Check sheet for the modelled part. Datum: model origin and axes. Units: mm. A direction names the side the tool comes from. Coordinates: 2 decimals unless noted, no trailing zeros. Loops run counter-clockwise (first coordinate to the right, second up) from the corner with the lowest first, then second, coordinate; pieces in that order, holes last. Notation, with made-up numbers: (60, 7) -> (112, 7) arc R26 ccw to (112, 43) -> close; hole circle Ø4 at (-3, 31). An arc over 180 degrees is marked (long way). Use CSV: the item, a comma, the result in double quotes.
```python
from build123d import *

# Parameters (mm, degrees)
SKETCH1_W           = 40
SKETCH1_H           = 50
BOSS_EXTRUDE1_DEPTH = 2
FILLET1_R           = 5
SKETCH2_R           = 1.25
CUT_EXTRUDE1_DEPTH  = 3
SKETCH3_W           = 40
SKETCH3_H           = 6
CUT_EXTRUDE3_DEPTH  = 3
BOSS_EXTRUDE2_DEPTH = 10
BOSS_EXTRUDE3_START = 10
BOSS_EXTRUDE3_DEPTH = 10
SKETCH7_R           = 6
CUT_EXTRUDE4_DEPTH  = 20
FILLET2_START       = 10
FILLET2_DEPTH       = 20


with BuildPart() as part:
    # Sketch1 → Boss-Extrude1 (new body)
    with BuildSketch(Plane.XY):
        with Locations((20, 25)):
            Rectangle(SKETCH1_W, SKETCH1_H)
    extrude(amount=BOSS_EXTRUDE1_DEPTH)

    # Fillet1
    fillet1_edges = [part.edges().sort_by_distance(p)[0] for p in [
        (0, 50, 1),
        (40, 50, 1),
    ]]
    fillet(fillet1_edges, radius=FILLET1_R)

    # Sketch2 → Cut-Extrude1 (cut)
    with BuildSketch(Plane.XY.offset(2)):
        with Locations((30.392304845, 19)):
            Circle(SKETCH2_R)
        with Locations((9.607695155, 19)):
            Circle(SKETCH2_R)
        with BuildLine():
            ThreePointArc((21.25, 37), (20.883883476, 37.883883476), (20, 38.25))
            Line((20, 38.25), (20, 35.75))
            ThreePointArc((20, 35.75), (20.883883476, 36.116116524), (21.25, 37))
        make_face()
        with BuildLine():
            Line((20, 35.75), (20, 38.25))
            ThreePointArc((20, 38.25), (18.75, 37), (20, 35.75))
        make_face()
    extrude(amount=-CUT_EXTRUDE1_DEPTH, mode=Mode.SUBTRACT)

    # Sketch3 → Cut-Extrude3 (cut)
    with BuildSketch(Plane.XY.offset(2)):
        with Locations((20, 3)):
            Rectangle(SKETCH3_W, SKETCH3_H)
    extrude(amount=-CUT_EXTRUDE3_DEPTH, mode=Mode.SUBTRACT)

    # Sketch5 → Boss-Extrude2 (add)
    with BuildSketch(Plane.ZY):
        with BuildLine():
            Line((3.77260129, 11.571238192), (4.515067527, 9.714158794))
            ThreePointArc((4.515067527, 9.714158794), (8.242796258, 9.312078644), (10, 6))
            ThreePointArc((10, 6), (6, 2), (2, 6))
            Line((2, 6), (0, 6))
            ThreePointArc((0, 6), (6, 0), (12, 6))
            ThreePointArc((12, 6), (9.364194387, 10.968117966), (3.77260129, 11.571238192))
        make_face()
    extrude(amount=-BOSS_EXTRUDE2_DEPTH)

    # Sketch6 → Boss-Extrude3 (add)
    with BuildSketch(Plane(origin=(40, 0, -40), x_dir=(0, 0, 1), z_dir=(-1, 0, 0)).offset(BOSS_EXTRUDE3_START)):
        with BuildLine():
            Line((43.77260129, 11.571238192), (44.515067527, 9.714158794))
            ThreePointArc((44.515067527, 9.714158794), (48.242796258, 9.312078644), (50, 6))
            ThreePointArc((50, 6), (46, 2), (42, 6))
            Line((42, 6), (40, 6))
            ThreePointArc((40, 6), (46, 0), (52, 6))
            ThreePointArc((52, 6), (49.364194387, 10.968117966), (43.77260129, 11.571238192))
        make_face()
    extrude(amount=-BOSS_EXTRUDE3_DEPTH)

    # Sketch7 → Cut-Extrude4 (cut)
    with BuildSketch(Plane(origin=(10, 0, 0), x_dir=(0, 0, -1), z_dir=(1, 0, 0))):
        with Locations((-6, 6)):
            Circle(SKETCH7_R)
    extrude(amount=CUT_EXTRUDE4_DEPTH, mode=Mode.SUBTRACT)

    # Fillet2: read off the stored shape, not the designer's step
    # Fillet2 outline → Fillet2 (cut)
    with BuildSketch(Plane.YZ.offset(FILLET2_START)):
        with BuildLine():
            Line((6, 0), (11.138093031, 0))
            ThreePointArc((11.138093031, 0), (10.1268882, 0.667027959), (10.342050449, 1.85915493))
            ThreePointArc((10.342050449, 1.85915493), (8.361665681, 0.484337283), (6, 0))
        make_face()
    extrude(amount=FILLET2_DEPTH, mode=Mode.SUBTRACT)


solid = part.part
```
1) Draft check along X on faces 1 (the cylindrical face through (31.547, 18.521, 1.014)), 2 (the cylindrical face through (39, 48, 1)), 3 (the flat face through (5, 11, 4)). Enter one of: released by +X, released by -X, zero draft, split by the parting line, or undercut.
Answer below:
face 1,"undercut"
face 2,"released by +X"
face 3,"zero draft"
2) Cross-section at D-D on y = 5. Record the boundary of the cut face in (x, z), and give its area (3 significant figures).
Answer below:
outline,"(0, 0.08) -> (10, 0.08) -> (10, 2.13) -> (0, 2.13) -> close; (0, 9.87) -> (10, 9.87) -> (10, 11.92) -> (0, 11.92) -> close; (30, 0.08) -> (40, 0.08) -> (40, 2.13) -> (30, 2.13) -> close; (30, 9.87) -> (40, 9.87) -> (40, 11.92) -> (30, 11.92) -> close"
area,"81.7 mm²"
3) Cross-section at A-A on y = 19. Record the boundary of the cut face in (x, z), and give its area (3 significant figures).
Answer below:
outline,"(0, 0) -> (8.36, 0) -> (8.36, 2) -> (0, 2) -> close; (10.86, 0) -> (29.14, 0) -> (29.14, 2) -> (10.86, 2) -> close; (31.64, 0) -> (40, 0) -> (40, 2) -> (31.64, 2) -> close"
area,"70.0 mm²"
4) Cross-section at B-B on z = 6. Record the boundary of the cut face in (x, y).
Answer below:
outline,"(0, 0) -> (10, 0) -> (10, 2) -> (0, 2) -> close; (0, 10) -> (10, 10) -> (10, 12) -> (0, 12) -> close; (30, 0) -> (40, 0) -> (40, 2) -> (30, 2) -> close; (30, 10) -> (40, 10) -> (40, 12) -> (30, 12) -> close"
5) Access from +Z, -Z, +X, -X, +Y, -Y to the whole of each face (thin tool, end or side, straight path). Record for faces 4 (the cylindrical face through (10.76, 18.52, 1.01)), 5 (the cylindrical face through (19.86, 10.134, 0.651)), 6 (the flat face through (35, 11, 4)).
Answer below:
face 4,"+Z, -Z"
face 5,"-Y"
face 6,"+X, -X"
6) Go/stop test with flat-tipped pins: pin 1 Ø1.5 at (x, y) = (9.61, 19) entering from -Z; pin 2 Ø5 at (y, z) = (9, 10.5) entering from -X; pin 3 Ø8 at (x, y) = (9, 25) entering from +Z. Record where each tip stops, or that it passes through.
Answer below:
pin 1,"passes through"
pin 2,"stops at x = 0"
pin 3,"stops at z = 2"
7) Cross-section at C-C on x = 27. Record the boundary of the cut face in (y, z).
Answer below:
outline,"(10.34, 1.86) arc R1.1 ccw to (11.14, 0) -> (50, 0) -> (50, 2) -> (10.47, 2) arc R6 cw to start"
8) Thickness scan on line 1 along Y through (x, z) = (8.5, 6.25); line 2 along Z through (x, y) = (28, 31); line 3 along Y through (x, z) = (5, 1.75). Record the ranges inside material, lowest first. Write a range as from..to.
Answer below:
line 1,"y = 0.01..2.01, 9.99..11.99"
line 2,"z = 0..2"
line 3,"y = 1.76..50"
